Verification items for the finished model (mm, model axes). A direction names the side the tool comes from. Give positions to 0.01 mm unless a question says otherwise; leave off trailing zeros. Order: outer loops, then holes, each group sorted by start corner. A loop starts at its lowest first (then second) coordinate and runs counter-clockwise, first axis right, second up.
from build123d import *

# Parameters (mm, degrees)
SKETCH1_W           = 7.9375
SKETCH1_H           = 7.9375
BOSS_EXTRUDE1_DEPTH = 4.2291
SKETCH2_W           = 5.3975
SKETCH2_H           = 5.3975
CUT_EXTRUDE1_DEPTH  = 7.1882
SKETCH3_R           = 2.69875
BOSS_EXTRUDE2_DEPTH = 1.397
SKETCH5_R           = 2.69875
BOSS_EXTRUDE4_DEPTH = 1.397
SKETCH6_R           = 1.5875
CUT_EXTRUDE2_DEPTH  = 11.7315


with BuildPart() as part:
    # Sketch1 → Boss-Extrude1 (new body, symmetric)
    with BuildSketch(Plane(origin=(0, 0, 0), x_dir=(1, 0, 0), z_dir=(0, 1, 0))):
        Rectangle(SKETCH1_W, SKETCH1_H)
    extrude(amount=BOSS_EXTRUDE1_DEPTH, both=True)

    # Sketch2 → Cut-Extrude1 (cut)
    with BuildSketch(Plane.XZ.offset(4.2291)):
        Rectangle(SKETCH2_W, SKETCH2_H)
    extrude(amount=-CUT_EXTRUDE1_DEPTH, mode=Mode.SUBTRACT)

    # Sketch3 → Boss-Extrude2 (add)
    with BuildSketch(Plane(origin=(0, 4.2291, 0), x_dir=(1, 0, 0), z_dir=(0, 1, 0))):
        Circle(SKETCH3_R)
    extrude(amount=BOSS_EXTRUDE2_DEPTH)

    # Sketch5 → Boss-Extrude4 (add)
    with BuildSketch(Plane(origin=(3.96875, 0, 0), x_dir=(0, 0, -1), z_dir=(1, 0, 0))):
        with Locations((0, 0.26035)):
            Circle(SKETCH5_R)
    boss_extrude4 = extrude(amount=BOSS_EXTRUDE4_DEPTH)

    # Mirror1: Boss-Extrude4 across plane
    add(boss_extrude4.mirror(Plane(origin=(0, 0, 0), x_dir=(0, 0, 1), z_dir=(1, 0, 0))))

    # Sketch6 → Cut-Extrude2 (cut, through all)
    with BuildSketch(Plane(origin=(5.36575, 0, 0), x_dir=(0, 0, -1), z_dir=(1, 0, 0))):
        with Locations((0, 0.26035)):
            Circle(SKETCH6_R)
    extrude(amount=-CUT_EXTRUDE2_DEPTH, mode=Mode.SUBTRACT)


solid = part.part
(1) Section check A-A, the plane z = 0. Enter the section's corners in (x, y).
Solved:
outline: (-5.37, -2.44) - (-3.97, -2.44) - (-3.97, -4.23) - (-2.7, -4.23) - (-2.7, -1.33) - (-5.37, -1.33) - close; (-5.37, 1.85) - (-2.7, 1.85) - (-2.7, 2.96) - (2.7, 2.96) - (2.7, 1.85) - (5.37, 1.85) - (5.37, 2.96) - (3.97, 2.96) - (3.97, 4.23) - (2.7, 4.23) - (2.7, 5.63) - (-2.7, 5.63) - (-2.7, 4.23) - (-3.97, 4.23) - (-3.97, 2.96) - (-5.37, 2.96) - close; (2.7, -4.23) - (3.97, -4.23) - (3.97, -2.44) - (5.37, -2.44) - (5.37, -1.33) - (2.7, -1.33) - close
(2) Scan lines: line 1 (X direction, y = -1.5, z = 0); line 2 (Z direction, x = 2.5, y = -1.75). Record each from-to range of solid material in increasing order.
Solved:
line 1: x = -5.37 to -2.7, 2.7 to 5.37
line 2: z = -3.97 to -2.7, 2.7 to 3.97
(3) Section check D-D, the plane z = 2. Enter the section's corners in (x, y), then the cut area to 3 significant figures.
Solved:
outline: (-5.37, -1.55) - (-3.97, -1.55) - (-3.97, -4.23) - (-2.7, -4.23) - (-2.7, 2.96) - (2.7, 2.96) - (2.7, -4.23) - (3.97, -4.23) - (3.97, -1.55) - (5.37, -1.55) - (5.37, 2.07) - (3.97, 2.07) - (3.97, 4.23) - (1.81, 4.23) - (1.81, 5.63) - (-1.81, 5.63) - (-1.81, 4.23) - (-3.97, 4.23) - (-3.97, 2.07) - (-5.37, 2.07) - close
area: 43.5 mm2
(4) Set-up check for faces 4 (the flat face through (0, -1, -2.699)), 5 (the flat face through (-3.969, -2, 2)), 6 (the cylindrical face through (-1.99, 4.92, -1.82)), 7 (the flat face through (3.969, -2, 2)): record each of +Z, -Z, +X, -X, +Y, -Y from which the full face is reachable in a straight line by a thin tool's end or side.
Solved:
face 4: -Y
face 5: -X
face 6: +Y
face 7: +X
(5) Section check B-B, the plane x = 0. Enter the section's corners in (y, z).
Solved:
outline: (-4.23, -3.97) - (4.23, -3.97) - (4.23, -2.7) - (5.63, -2.7) - (5.63, 2.7) - (4.23, 2.7) - (4.23, 3.97) - (-4.23, 3.97) - (-4.23, 2.7) - (2.96, 2.7) - (2.96, -2.7) - (-4.23, -2.7) - close
(6) Release check for a two-part mould opening along Z. For faces 1 (the flat face through (2.699, -1.5, 0)), 2 (the cylindrical face through (4.657, -1.382, 2.142)), 3 (the flat face through (-5.366, -2, 0)) record: pulls with the +Z half, pulls with the -Z half, needs draft (parallel to the pull), parting line crosses it, or undercut.
Solved:
face 1: undercut
face 2: parting line crosses it
face 3: needs draft
(7) Section check C-C, the plane x = -3.75. Enter the section's corners in (y, z) (1 decimal).
Solved:
outline: (-4.2, -4) - (4.2, -4) - (4.2, 4) - (-4.2, 4) - close; hole circle Ø3.2 at (0.3, 0)
(8) Go/stop test with flat-tipped pins: pin 1 (1.5 mm diameter, centred on y = 3.5, z = -2.5, fed in from +X); pin 2 (1.6 mm diameter, centred on x = -1, z = -1, fed in from -Y). Record where each tip stops, or that it passes through.
Solved:
pin 1: stops at x = 3.97
pin 2: stops at y = 2.96
